Can you work these out from the model? Positions are in its coordinate system, mm. A direction names the side the tool comes from. Give positions to 0.01 mm unless a question says otherwise; leave off trailing zeros. Order: outer loops, then holes, each group sorted by start corner. A loop starts at its lowest first (then second) coordinate and runs counter-clockwise, first axis right, second up.
```python
from build123d import *

# Parameters (mm, degrees)
SKETCH1_W           = 45
SKETCH1_H           = 26
BOSS_EXTRUDE1_DEPTH = 18
SKETCH2_W           = 48
SKETCH2_H           = 29
SKETCH2_W_2         = 35.8
SKETCH2_H_2         = 18
BOSS_EXTRUDE2_DEPTH = 3
CHAMFER1_SIZE       = 1
CHAMFER2_SIZE       = 4
CHAMFER2_SIZE2      = 2.309401077


with BuildPart() as part:
    # Sketch1 → Boss-Extrude1 (new body)
    with BuildSketch(Plane(origin=(0, 0, 0), x_dir=(1, 0, 0), z_dir=(0, 1, 0))):
        Rectangle(SKETCH1_W, SKETCH1_H)
    extrude(amount=BOSS_EXTRUDE1_DEPTH)

    # Sketch2 → Boss-Extrude2 (add)
    with BuildSketch(Plane(origin=(0, 18, 0), x_dir=(1, 0, 0), z_dir=(0, 1, 0))):
        Rectangle(SKETCH2_W, SKETCH2_H)
        Rectangle(SKETCH2_W_2, SKETCH2_H_2, mode=Mode.SUBTRACT)
    extrude(amount=BOSS_EXTRUDE2_DEPTH)

    # Chamfer1
    chamfer1_edges = [part.edges().sort_by_distance(p)[0] for p in [
        (24, 21, 0),
        (0, 21, -14.5),
        (-24, 21, 0),
        (0, 21, 14.5),
    ]]
    chamfer(chamfer1_edges, length=CHAMFER1_SIZE)

    # Chamfer2
    chamfer2_edges = [part.edges().sort_by_distance(p)[0] for p in [
        (17.9, 21, 0),
        (0, 21, -9),
        (-17.9, 21, 0),
        (0, 21, 9),
    ]]
    chamfer2_side = [part.faces().sort_by_distance(p)[0] for p in [
        (22.466614586, 21, 0),
    ]]
    chamfer(chamfer2_edges, length=CHAMFER2_SIZE, length2=CHAMFER2_SIZE2, reference=chamfer2_side[0])


solid = part.part
```
1) We'd pull the mould along X, two halves only. Please class faces 1 (the face through (-23.5, 20.5, 0.2)), 2 (the face through (19.87, 19.83, 0.18)), 3 (the face through (-0.3, 20.5, -14)): +X half, -X half, draft (parallel to the pull), parting line (faces both ways), or undercut.
2) Suppose I cut it at A-A (x = -16). Please give me the cut outline in (y, z), and give its area (3 significant figures).
3) Suppose I cut it at B-B (z = -4). Please give me the cut outline in (x, y), and give its area (3 significant figures).
4) If I drill on line 1 (X direction, y = 18.5, z = -3.5); line 2 (X direction, y = 7.5, z = 12); line 3 (Y direction, x = -12.5, z = 7.75), over which ranges is the centre line in solid material (lowest first)?
5) Which directions (+Z, -Z, +X, -X, +Y, -Y) give clear straight access to the entire face, cutting with the end or side of a thin tool? Please do faces 4 (the face through (0, 0, 0)), 5 (the face through (-22.5, 9, 0)), 6 (the face through (0, 18, 0)), 7 (the face through (0, 9, 13)), 8 (the face through (22.5, 9, 0)).
6) Suppose I cut it at C-C (y = 11.5). Please give me the cut outline in (x, z).
7) Suppose I cut it at D-D (z = -9.5). Please give me the cut outline in (x, y), and give its area (3 significant figures).
8) I'm going to push flat-ended pins straight in: pin 1 Ø5.5 at (y, z) = (8, -5.5) entering from -X; pin 2 Ø5.5 at (x, y) = (-11, 11) entering from +Z; pin 3 Ø6 at (x, z) = (-16.5, 6) entering from +Y. Where does each tip first touch, or does it pass through?
Results:
1. face 1: -X half
1. face 2: undercut
1. face 3: draft
2. outline: (0, -13) - (18, -13) - (18, -14.5) - (20, -14.5) - (21, -13.5) - (21, -13) - (18.69, -9) - (18, -9) - (18, 9) - (18.69, 9) - (21, 13) - (21, 13.5) - (20, 14.5) - (18, 14.5) - (18, 13) - (0, 13) - close
2. area: 491 mm2
3. outline: (-24, 18) - (-22.5, 18) - (-22.5, 0) - (22.5, 0) - (22.5, 18) - (24, 18) - (24, 20) - (23, 21) - (21.9, 21) - (17.9, 18.69) - (17.9, 18) - (-17.9, 18) - (-17.9, 18.69) - (-21.9, 21) - (-23, 21) - (-24, 20) - close
3. area: 836 mm2
4. line 1: x = -24 to -17.9, 17.9 to 24
4. line 2: x = -22.5 to 22.5
4. line 3: y = 0 to 18
5. face 4: +Z, -Z, +X, -X, -Y
5. face 5: +Z, -Z, -X, -Y
5. face 6: +Y
5. face 7: +Z, +X, -X, -Y
5. face 8: +Z, -Z, +X, -Y
6. outline: (-22.5, -13) - (22.5, -13) - (22.5, 13) - (-22.5, 13) - close
7. outline: (-24, 18) - (-22.5, 18) - (-22.5, 0) - (22.5, 0) - (22.5, 18) - (24, 18) - (24, 20) - (23, 21) - (21.9, 21) - (18.4, 18.98) - (-18.4, 18.98) - (-21.9, 21) - (-23, 21) - (-24, 20) - close
7. area: 872 mm2
8. pin 1: stops at x = -22.5
8. pin 2: stops at z = 13
8. pin 3: stops at y = 19.61
